Could you check a few things on this model? Use its own coordinates, in mm. Face numbers are marked on the shaded views. A direction names the side the tool comes from. Give positions to 0.01 mm unless a question says otherwise; leave off trailing zeros. Loops run counter-clockwise (first coordinate to the right, second up) from the corner with the lowest first, then second, coordinate; pieces in that order, holes last. Notation, with made-up numbers: M 17,-7.5 L 45,-7.5 A9 cw 45,-3.5 Z; hole C 59,-24 d6. An arc over 180 degrees is marked long. Return JSON: item names as keys, results as strings. Group by question number.
1. If we section it at C-C (z = 12.5): Write out the boundary of the cut face in (x, y).
2. If we section it at A-A (y = 82): Write out the boundary of the cut face in (x, z).
3. For the marked faces 1, 2 and 3, which set-ups out of +Z, -Z, +X, -X, +Y, -Y let a thin tool reach every point of the face, with its end or its side?
4. If we section it at B-B (x = 98): Write out the boundary of the cut face in (y, z), plus the area to 3 significant figures.
5. For pin 1 (4 mm diameter, centred on y = 5.5, z = 17.5, fed in from +X); pin 2 (2.5 mm diameter, centred on y = 5.5, z = 8.5, fed in from -X); pin 3 (6.5 mm diameter, centred on x = 4.5, z = 14, fed in from +Y); pin 4 (3 mm diameter, centred on x = 98, y = 82, fed in from +Z), each with a flat end and sliding along its axis, tell me the tip position at first contact or that it passes through.
6. Please list where these lines run through material, in increasing order: line 1 (Y direction, x = 4, z = 1.25); line 2 (X direction, y = 4, z = 0.95).
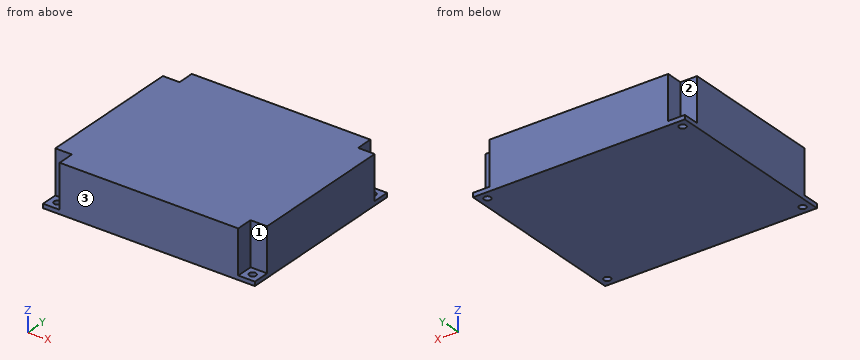
Solid Edge part; units mm, degrees
sketch "Sketch1" plane through (0, 0, 0) normal (0, 0, 1) x (1, 0, 0)
  line L0 (0, 0) -> (102, 0)
  line L1 (102, 0) -> (102, 86)
  line L2 (102, 86) -> (0, 86)
  line L3 (0, 86) -> (0, 0)
extrude "Protrusion1" add sketch "Sketch1" along normal blind 23
sketch "Sketch2" plane through (51, 43, 23) normal (0, 0, 1) x (1, 0, 0)
  circle A0 centre (-47, 39) radius 1.65
extrude "ExtrudedCutout_1" cut sketch "Sketch2" against normal blind 23
mirror "Mirror1" about plane through (51, 43, 11.5) normal (0, -1, 0) of "ExtrudedCutout_1"
mirror "Mirror2" about plane through (51, 43, 11.5) normal (1, 0, 0) of "ExtrudedCutout_1", "Mirror1"
sketch "Sketch3" plane through (51, 43, 23) normal (0, 0, 1) x (1, 0, 0)
  line L0 (-51, -43) -> (-43, -43)
  line L1 (-43, -43) -> (-43, -35)
  line L2 (-43, -35) -> (-51, -35)
  line L3 (-51, -35) -> (-51, -43)
  line L4 (51, 43) -> (43, 43)
  line L5 (43, 43) -> (43, 35)
  line L6 (43, 35) -> (51, 35)
  line L7 (51, 35) -> (51, 43)
  line L8 (51, -43) -> (51, -35)
  line L9 (51, -35) -> (43, -35)
  line L10 (43, -35) -> (43, -43)
  line L11 (43, -43) -> (51, -43)
  line L12 (-51, 43) -> (-51, 35)
  line L13 (-51, 35) -> (-43, 35)
  line L14 (-43, 35) -> (-43, 43)
  line L15 (-43, 43) -> (-51, 43)
extrude "ExtrudedCutout_2" cut sketch "Sketch3" against normal blind 21
Answer:
{
 "1": {"outline": "M 0,8 L 8,8 L 8,0 L 94,0 L 94,8 L 102,8 L 102,78 L 94,78 L 94,86 L 8,86 L 8,78 L 0,78 Z"},
 "2": {"outline": "M 0,0 L 2.35,0 L 2.35,2 L 0,2 Z; M 5.65,0 L 96.35,0 L 96.35,2 L 94,2 L 94,23 L 8,23 L 8,2 L 5.65,2 Z; M 99.65,0 L 102,0 L 102,2 L 99.65,2 Z"},
 "3": {"face 1": "+Z, +X, -Y", "face 2": "+Z, -X, +Y", "face 3": "+Z, -Z, +X, -X, -Y"},
 "4": {"outline": "M 0,0 L 2.35,0 L 2.35,2 L 0,2 Z; M 5.65,0 L 80.35,0 L 80.35,2 L 78,2 L 78,23 L 8,23 L 8,2 L 5.65,2 Z; M 83.65,0 L 86,0 L 86,2 L 83.65,2 Z", "area": "1,630 mm²"},
 "5": {"pin 1": "stops at x = 94", "pin 2": "stops at x = 8", "pin 3": "stops at y = 78", "pin 4": "passes through"},
 "6": {"line 1": "y = 0 to 2.35, 5.65 to 80.35, 83.65 to 86", "line 2": "x = 0 to 2.35, 5.65 to 96.35, 99.65 to 102"}
}
